Part model, mm, in its own coordinate system. Face numbers are marked on the shaded views. Coordinates: 2 decimals unless noted, no trailing zeros. Loops run counter-clockwise (first coordinate to the right, second up) from the corner with the lowest first, then second, coordinate; pieces in that order, holes last. Notation, with made-up numbers: (-22, -33.5) - (-10, -33.5) arc R35 cw to (-10, -0.5) - close; hole circle Ø10 at (44.25, -28.5). An arc over 180 degrees is marked (long way). Answer as CSV lines item,"result".
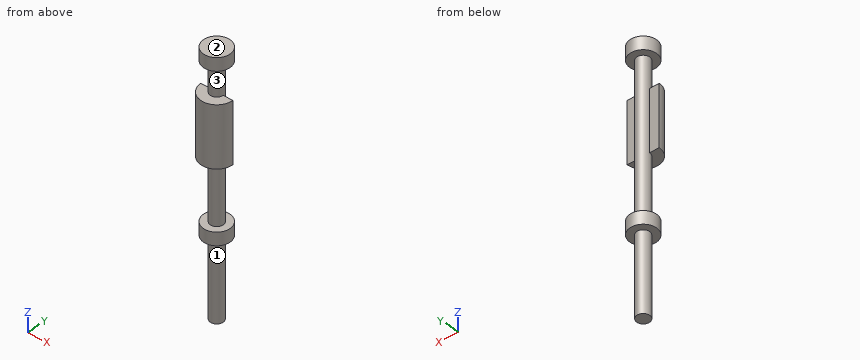
Autodesk Inventor part; units mm, degrees
ref_plane "YZ Plane" through (0, 0, 0) normal (1, 0, 0) x (0, 1, 0)
ref_plane "XZ Plane" through (0, 0, 0) normal (0, 1, 0) x (-1, 0, 0)
ref_plane "XY Plane" through (0, 0, 0) normal (0, 0, 1) x (1, 0, 0)
sketch "Эскиз1" plane through (0, 0, 0) normal (0, 0, 1) x (1, 0, 0)
  circle A0 centre (0, 0) radius 8.5
  dimension "d1" = 17
extrude "Выдавливание1" add sketch "Эскиз1" against normal blind 55
sketch "Эскиз2" plane through (0, 0, 0) normal (0, 0, 1) x (1, 0, 0)
  circle A0 centre (0, 0) radius 8.5
  dimension "d10" = 17
extrude "Выдавливание2" add sketch "Эскиз2" along normal blind 30
sketch "Эскиз3" plane through (0, 0, 30) normal (0, 0, 1) x (1, 0, 0)
  circle A0 centre (0, 0) radius 17.5
  dimension "d7" = 35
extrude "Выдавливание3" add sketch "Эскиз3" along normal blind 17
sketch "Эскиз4" plane through (0, 0, 47) normal (0, 0, 1) x (1, 0, 0)
  circle A0 centre (0, 0) radius 8.5
  line L0 (8.5, 0) -> (20, 0)
  point P0 (-16, 0)
  dimension "d25" = 17
extrude "Выдавливание4" add sketch "Эскиз4" along normal blind 15
sketch "Эскиз6" plane through (0, 0, 62) normal (0, 0, 1) x (1, 0, 0)
  circle A0 centre (0, 0) radius 8.5
  point P0 (-16, 0)
  point P1 (20, 0)
  dimension "d24" = 17
extrude "Выдавливание5" add sketch "Эскиз6" along normal blind 55
sketch "Эскиз7" plane through (0, 0, 117) normal (0, 0, 1) x (1, 0, 0)
  circle A0 centre (0, 0) radius 8.5
  dimension "d26" = 17
extrude "Выдавливание6" add sketch "Эскиз7" along normal blind 130
sketch "Эскиз8" plane through (0, 0, 247) normal (0, 0, 1) x (1, 0, 0)
  circle A0 centre (0, 0) radius 17.5
  dimension "d23" = 35
extrude "Выдавливание7" add sketch "Эскиз8" along normal blind 17
sketch "Эскиз9" plane through (0, 0, -55) normal (0, 0, -1) x (-1, 0, 0)
  circle A0 centre (0, 0) radius 8.5
extrude "Выдавливание8" add sketch "Эскиз9" along normal blind 19.1
ref_plane "РабПлоскость1" through (0, 0, 168) normal (0, 0, 1) x (1, 0, 0)
sketch "Эскиз10" plane through (0, 0, 168) normal (0, 0, 1) x (1, 0, 0)
  circle A0 centre (0, 0) radius 8.5
  circle A1 centre (0, 0) radius 21
  line L0 (-21, 0) -> (21, 0)
  point P0 (-8.5, 0)
  point P1 (8.5, 0)
  dimension "d30" = 42
extrude "Выдавливание9" add sketch "Эскиз10" along normal mid plane 80 contours L0 A1 A0 picked at (16.6299, -1.6752)
properties part number "балансирный_вал"
Q1. Saw through at D-D (z = 148.5). Give the cut face in (x, y).
Results:
outline,"(-21, 0) arc R21 ccw to (21, 0) - (8.5, 0) arc R8.5 ccw to (-8.5, 0) - close"
Q2. Saw through at B-B (y = -11.5). Give the cut face in (x, z).
Results:
outline,"(-17.57, 128) - (17.57, 128) - (17.57, 208) - (-17.57, 208) - close; (-13.19, 30) - (13.19, 30) - (13.19, 47) - (-13.19, 47) - close; (-13.19, 247) - (13.19, 247) - (13.19, 264) - (-13.19, 264) - close"
Q3. Saw through at C-C (y = 12). Give the cut face in (x, z), then the cut area to 3 significant figures.
Results:
outline,"(-12.74, 30) - (12.74, 30) - (12.74, 47) - (-12.74, 47) - close; (-12.74, 247) - (12.74, 247) - (12.74, 264) - (-12.74, 264) - close"
area,"866 mm^2"
Q4. Wall check: L1, parallel to Z at x = 2, y = -11.5; L2, parallel to Z at x = 0, y = 11.5; L3, parallel to Z at x = 17, y = -5.5. Give the ranges that are in metal, low to high.
Results:
L1,"z = 30 to 47, 128 to 208, 247 to 264"
L2,"z = 30 to 47, 247 to 264"
L3,"z = 128 to 208"
Q5. Two-plate mould, pull along Z, no slides. Class the marked faces 1, 2 and 3: released by +Z, released by -Z, zero draft, split by the parting line, or undercut.
Results:
face 1,"zero draft"
face 2,"released by +Z"
face 3,"undercut"
Q6. Saw through at A-A (x = 0). Give the cut face in (y, z).
Results:
outline,"(-21, 128) - (-8.5, 128) - (-8.5, 47) - (-17.5, 47) - (-17.5, 30) - (-8.5, 30) - (-8.5, -74.1) - (8.5, -74.1) - (8.5, 30) - (17.5, 30) - (17.5, 47) - (8.5, 47) - (8.5, 247) - (17.5, 247) - (17.5, 264) - (-17.5, 264) - (-17.5, 247) - (-8.5, 247) - (-8.5, 208) - (-21, 208) - close"
Q7. Flat gauge pins, fed straight in: pin 1 (12 mm diameter, centred on x = 15.5, z = 26, fed in from -Y); pin 2 (1 mm diameter, centred on y = 8, z = -5.5, fed in from +X); pin 3 (10 mm diameter, centred on y = -9, z = 204.5, fed in from +X). Where does each tip first touch, or does it go through?
Results:
pin 1,"stops at y = -13.59"
pin 2,"stops at x = 4"
pin 3,"stops at x = 20.62"
